```python
from build123d import *

# Parameters (mm, degrees)
F1_DEPTH    = 2
F2_T1_DEPTH = 27.7168298797


# Not quite as in the source:
# - a fillet or chamfer that OpenCascade refuses, or shapes differently, is made with other operations: its cross-section is extruded or revolved along the edge and cut away or added


with BuildPart() as f1:
    # F0 (on Front) → F1 (new body)
    with BuildSketch(Plane.XZ):
        with BuildLine():
            Line((38.9543399215, 33.578529954), (46.6473846136, 4.5816842054))
            Line((46.6473846136, 4.5816842054), (47.6139461386, 4.8381190285))
            Line((47.6139461386, 4.8381190285), (39.9209014464, 33.834964777))
            Line((39.9209014464, 33.834964777), (39.9209014464, 34.991762988))
            add(Edge.make_bspline(
                [(38.9543399215, 33.578529954), (39.261396009, 34.083414355), (39.5680450127, 34.5875702619), (39.9209014464, 34.991762988)],
                knots=[0, 0, 0, 0, 0.0840395323, 0.0840395323, 0.0840395323, 0.0840395323], degree=3))
        make_face()
        with BuildLine():
            add(Edge.make_bspline(
                [(38.9543399215, 33.578529954), (37.6640439923, 34.1443154), (34.8932435121, 35.3619439278), (32.5863528285, 29.9762581485), (26.5655761049, 32.3528079023), (26.8476535004, 30.0684064483), (26.7979316413, 29.2242113501)],
                knots=[0, 0, 0, 0, 0.2516937882, 0.52851586, 0.8089732942, 1, 1, 1, 1], degree=3))
            add(Edge.make_bspline(
                [(38.9543399215, 33.578529954), (39.261396009, 34.083414355), (39.5680450127, 34.5875702619), (39.9209014464, 34.991762988)],
                knots=[0, 0, 0, 0, 0.0840395323, 0.0840395323, 0.0840395323, 0.0840395323], degree=3))
            add(Edge.make_bspline(
                [(39.9209014464, 34.991762988), (40.305091024, 35.4318474469), (40.7440586925, 35.7534273237), (41.2979722023, 35.8284153044)],
                knots=[0.0840395323, 0.0840395323, 0.0840395323, 0.0840395323, 0.1755416542, 0.1755416542, 0.1755416542, 0.1755416542], degree=3))
            add(Edge.make_bspline(
                [(41.2979722023, 35.8284153044), (41.4906721415, 35.8545027334), (41.6972835341, 35.850746093), (41.914248864, 35.8273036468)],
                knots=[0.1755416542, 0.1755416542, 0.1755416542, 0.1755416542, 0.2073741569, 0.2073741569, 0.2073741569, 0.2073741569], degree=3))
            add(Edge.make_bspline(
                [(41.914248864, 35.8273036468), (43.1236682433, 35.696629549), (46.5485390265, 34.0361170247), (48.7293844979, 38.5978142218), (50.4905452243, 38.5674441057), (50.8079711977, 38.5090563461)],
                knots=[0.2073741569, 0.2073741569, 0.2073741569, 0.2073741569, 0.3848165425, 0.6042792737, 0.6509015915, 0.6509015915, 0.6509015915, 0.6509015915], degree=3))
            Line((50.8079711977, 38.5090563461), (49.6484453004, 39.2675593609))
            Line((49.6484453004, 39.2675593609), (36.1188769209, 48.1179165882))
            Line((36.1188769209, 48.1179165882), (36.6174241261, 48.182718962))
            Line((36.6174241261, 48.182718962), (57.1271326119, 38.8518427461))
            Line((57.1271326119, 38.8518427461), (57.7971301973, 38.5470278562))
            Line((57.7971301973, 38.5470278562), (58.3644174039, 39.0885546803))
            Line((58.3644174039, 39.0885546803), (36.2102526821, 49.1675750053))
            Line((36.2102526821, 49.1675750053), (34.7956053054, 52.5892884836))
            Line((34.7956053054, 52.5892884836), (33.3790388766, 52.9607144486))
            Line((33.3790388766, 52.9607144486), (34.0435805037, 47.848164531))
            Line((34.0435805037, 47.848164531), (21.2916761887, 29.0061510308))
            add(Edge.make_bspline(
                [(21.2916761887, 29.0061510308), (22.2377144422, 29.3003004789), (24.1919394004, 29.7248092747), (25.9431803037, 29.402753862), (26.7979316413, 29.2242113501)],
                knots=[0, 0, 0, 0, 0.5149489736, 1, 1, 1, 1], degree=3))
        make_face()
        with BuildLine():
            Line((35.3305023149, 48.0154417465), (27.6333307537, 32.0162793804))
            add(Edge.make_bspline(
                [(22.623414625, 30.0818228404), (23.0984624572, 30.271051787), (24.0718553407, 30.6285749561), (26.4700247065, 29.5668028622), (26.2229246754, 31.0093421737), (27.2691634193, 31.7917195395), (27.4724411863, 32.0150673015), (27.6333307537, 32.0162793804)],
                knots=[0, 0, 0, 0, 0.2344131875, 0.4959636953, 0.6719941358, 0.8783364267, 1, 1, 1, 1], degree=3))
            Line((22.623414625, 30.0818228404), (34.4592127341, 47.5702122015))
            Line((34.4592127341, 47.5702122015), (34.6295802641, 47.9243341999))
            Line((34.6295802641, 47.9243341999), (35.3305023149, 48.0154417465))
        make_face(mode=Mode.SUBTRACT)
        with BuildLine():
            add(Edge.make_bspline(
                [(28.1314488439, 31.9244866572), (28.7524146036, 31.8044131569), (30.0444740365, 31.5255182244), (31.7027687342, 31.5518548648), (32.4930864971, 32.4035579454), (32.8194445517, 33.3447504689), (33.7630925871, 34.2287315693), (34.7377791878, 34.5605212888), (35.1689763006, 34.6552392698), (35.3122933345, 34.7550361976)],
                knots=[0.0420238635, 0.0420238635, 0.0420238635, 0.0420238635, 0.1988600446, 0.3671317013, 0.4980303245, 0.6259677195, 0.7707900684, 0.901825209, 1, 1, 1, 1], degree=3))
            Line((28.1314488439, 31.9244866572), (35.3289500731, 46.8850458548))
            Line((35.3289500731, 46.8850458548), (35.3122933345, 34.7550361976))
        make_face(mode=Mode.SUBTRACT)
        with BuildLine():
            Line((35.7789325262, 47.0996380734), (41.0592946479, 36.3158529826))
            add(Edge.make_bspline(
                [(35.8884423072, 34.9503078622), (36.4754899607, 34.9773776718), (37.5532358859, 34.9460992821), (38.8819756802, 33.9391375769), (39.5472460755, 35.7321102048), (40.3992507331, 36.2208948371), (41.0592946479, 36.3158529826)],
                knots=[0, 0, 0, 0, 0.2672899311, 0.493356995, 0.7378410778, 1, 1, 1, 1], degree=3))
            Line((35.8884423072, 34.9503078622), (35.7789325262, 47.0996380734))
        make_face(mode=Mode.SUBTRACT)
        Polygon((35.8180012475, 48.678030682), (34.5529859469, 48.5136009278), (34.0623831223, 52.2879791273), (34.5787238251, 52.1228960279), align=None, mode=Mode.SUBTRACT)
        with BuildLine():
            add(Edge.make_bspline(
                [(41.6765891777, 36.3158529826), (42.8641978584, 36.0833171062), (44.6938094993, 35.7263694764), (45.6901446165, 35.8578817285), (47.6400405781, 37.6167605803), (48.6840130278, 38.4955786117), (49.1976533289, 38.9442550866)],
                knots=[0, 0, 0, 0, 0.305073377, 0.4728149529, 0.7460971216, 1, 1, 1, 1], degree=3))
            Line((41.6765891777, 36.3158529826), (36.2907871604, 47.3872721195))
            Line((36.2907871604, 47.3872721195), (49.1976533289, 38.9442550866))
        make_face(mode=Mode.SUBTRACT)
        with BuildLine():
            Line((49.6484453004, 39.2675593609), (50.8079711977, 38.5090563461))
            add(Edge.make_bspline(
                [(50.8079711977, 38.5090563461), (51.8830810784, 38.3112991915), (54.484160752, 36.5282918381), (56.6203789239, 37.8247061914), (57.7971301973, 38.5470278562)],
                knots=[0.6509015915, 0.6509015915, 0.6509015915, 0.6509015915, 0.8088096356, 1, 1, 1, 1], degree=3))
            Line((57.7971301973, 38.5470278562), (57.1271326119, 38.8518427461))
            add(Edge.make_bspline(
                [(49.6484453004, 39.2675593609), (50.3456305804, 39.2010948295), (51.7025455015, 39.0717365126), (53.4260999906, 38.2284905671), (54.784884825, 37.8599443173), (56.2669250792, 38.487560835), (57.1271326119, 38.8518427461)],
                knots=[0, 0, 0, 0, 0.2603727588, 0.5067572303, 0.7137114564, 1, 1, 1, 1], degree=3))
        make_face()
    extrude(amount=F1_DEPTH)

    # F2: chamfer of 5 on 1 edges, made by hand

    # F2_s2 → F2_t1 (cut)
    with BuildSketch(Plane.XZ.offset(-12.8584149398)):
        Polygon((45.3652104983, 9.4144918302), (51.4801922384, 5.8638583208), (46.6473846136, 4.5816842054), align=None)
    extrude(amount=F2_T1_DEPTH, mode=Mode.SUBTRACT)


solid = f1.part
```
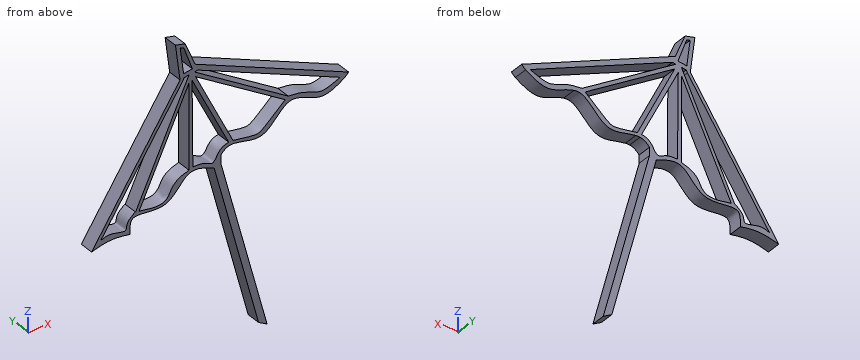
Could you check a few things on this model? Use its own coordinates, in mm. Round coordinates to 2 decimals unless told otherwise and drop trailing zeros. Loops run counter-clockwise (first coordinate to the right, second up) from the corner with the lowest first, then second, coordinate; pieces in that order, holes last.
Q1. I want a section at A-A (z = 44.5). Write out the boundary of the cut face in (x, y), and give its area (3 significant figures).
Q2. I want a section at D-D (z = 20). Write out the boundary of the cut face in (x, y), and give its area (3 significant figures).
Q3. Please list where these lines run through material, in increasing order: L1, parallel to Z at x = 30, y = -1; L2, parallel to X at y = -0.6, z = 46; L3, parallel to X at y = -1.7, z = 46.5.
Q4. For P1, Ø1, axis at y = -1.5, z = 38, coming from the -X side; P2, Ø0.6, axis at y = -1, z = 34.5, coming from the +X side, each with a flat end and sliding along its axis, tell me the tip position at first contact or that it passes through.
Q5. I want a section at B-B (x = 32). Give the number of separate pieces and of enclosed holes in the cut face, and give its area (3 significant figures).
Answer below:
1. outline: (31.78, -2) - (32.38, -2) - (32.38, 0) - (31.78, 0) - close; (33.64, -2) - (34.18, -2) - (34.18, 0) - (33.64, 0) - close; (35.33, -2) - (35.8, -2) - (35.8, 0) - (35.33, 0) - close; (37.05, -2) - (37.7, -2) - (37.7, 0) - (37.05, 0) - close; (40.7, -2) - (41.65, -2) - (41.65, 0) - (40.7, 0) - close; (44.71, -2) - (46.47, -2) - (46.47, 0) - (44.71, 0) - close
1. area: 9.94 mm2
2. outline: (42.56, -2) - (43.59, -2) - (43.59, 0) - (42.56, 0) - close
2. area: 2.07 mm2
3. L1: z = 31.23 to 31.6, 35.81 to 36.94, 40.98 to 41.87
3. L2: x = 32.79 to 33.4, 34.36 to 34.9, 35.33 to 35.79, 36.32 to 36.97, 38.41 to 39.36, 41.42 to 43.17
3. L3: x = 33.13 to 33.73, 34.6 to 35.14, 35.33 to 35.78, 36.07 to 36.72, 37.65 to 38.59, 40.32 to 42.07
4. P1: stops at x = 27.04
4. P2: stops at x = 39.92
5. separate pieces: 3
5. enclosed holes: 0
5. area: 5.12 mm2
